Geometry: final body of the model. Coordinates: model frame, mm. A direction names the side the tool comes from. Coordinates: 2 decimals unless noted, no trailing zeros. Order: outer loops, then holes, each group sorted by start corner. A loop starts at its lowest first (then second) coordinate and runs counter-clockwise, first axis right, second up. Notation, with made-up numbers: (77, 32.25) -> (86, 32.25) arc R19 cw to (86, 38.25) -> close; hole circle Ø10 at (-26.5, 74.25). An arc over 180 degrees is marked (long way). Answer in a Markdown table with one row per item. Add a question column.
1) Section query A-A on y = 19.5. Return the cut outline in (x, z).
2) Contact query for flat-ended pins moving along their axis: P1, Ø8, axis at x = 9, z = 41.5, coming from the +Y side; P2, Ø11, axis at x = 16, z = 33.5, coming from the -Y side; P3, Ø2, axis at x = 10, y = 4.5, coming from the -Z side. Output: stop coordinate, or through.
3) Set-up query: faces 1 (the face through (11.63, -2.46, 38.1)), 2 (the face through (11, 2, 23)), 3 (the face through (21.5, 14, 24)). Return all of +Z, -Z, +X, -X, +Y, -Y with unobstructed straight access to the full face (end or side cutting, diameter ignored); none if empty.
4) Ray query, line 1 (X direction, y = 17.5, z = 27); line 2 (Y direction, x = 9, z = 37); line 3 (Z direction, x = 9.25, y = 21). Return the intervals inside material, ascending. Write a range as from..to.
5) Pull-direction query (Z, two-part tool) for faces 4 (the face through (1, 12, 0)), 5 (the face through (11.63, -2.46, 8.1)), 6 (the face through (11, 14, 48.5)), 7 (the face through (11, -5, 9)); classes: +Z half, -Z half, draft (parallel to the pull), parting line (faces both ways), or undercut.
6) Section query D-D on x = 3. Return the cut outline in (y, z).
7) Section query B-B on x = 10.75. Return the cut outline in (y, z), then the cut area to 3 significant figures.
8) Section query C-C on z = 39.25. Return the cut outline in (x, y).
```python
from build123d import *

# Parameters (mm, degrees)
SKETCH2_W           = 21.5
SKETCH2_H           = 28.5
BOSS_EXTRUDE6_DEPTH = 48.5
CUT_EXTRUDE5_DEPTH  = 46.5
SKETCH5_R           = 1.45
BOSS_EXTRUDE7_DEPTH = 5


with BuildPart() as part:
    # Sketch2 → Boss-Extrude6 (new body)
    with BuildSketch(Plane.XY):
        with Locations((10.75, 14.25)):
            Rectangle(SKETCH2_W, SKETCH2_H)
    extrude(amount=BOSS_EXTRUDE6_DEPTH)

    # 3DSketch6 → Cut-Extrude5 (cut)
    with BuildSketch(Plane(origin=(19.5, 2, 0), x_dir=(-0.5510615347417098, 0.8344646097517326, 0), z_dir=(0, 0, 1))):
        Polygon((0, 0), (22.113312158, -14.603130671), (31.756889016, 0), (9.643576858, 14.603130671), align=None)
    extrude(amount=CUT_EXTRUDE5_DEPTH, mode=Mode.SUBTRACT)

    # Sketch5 → Boss-Extrude7 (add)
    with BuildSketch(Plane(origin=(0, 0, 0), x_dir=(-1, 0, 0), z_dir=(0, -1, 0))):
        with Locations(Location((-10.75, -39.25, 0), (0, 0, 270))):
            Circle(SKETCH5_R)
        with Locations(Location((-10.75, -9.25, 0), (0, 0, 270))):
            Circle(SKETCH5_R)
    extrude(amount=BOSS_EXTRUDE7_DEPTH)


solid = part.part
```
Result:
| question | item | result |
|---|---|---|
| 1 | outline | (0, 0) -> (2, 0) -> (2, 46.5) -> (19.5, 46.5) -> (19.5, 0) -> (21.5, 0) -> (21.5, 48.5) -> (0, 48.5) -> close |
| 2 | P1 | y = 2 |
| 2 | P2 | y = 0 |
| 2 | P3 | z = 46.5 |
| 3 | face 1 | -Y |
| 3 | face 2 | -Z, +Y |
| 3 | face 3 | +Z, -Z, +X, +Y, -Y |
| 4 | line 1 | 0..2, 19.5..21.5 |
| 4 | line 2 | 0..2 |
| 4 | line 3 | 46.5..48.5 |
| 5 | face 4 | -Z half |
| 5 | face 5 | undercut |
| 5 | face 6 | +Z half |
| 5 | face 7 | draft |
| 6 | outline | (0, 0) -> (2, 0) -> (2, 46.5) -> (28.5, 46.5) -> (28.5, 48.5) -> (0, 48.5) -> close |
| 7 | outline | (-5, 7.8) -> (0, 7.8) -> (0, 0) -> (2, 0) -> (2, 46.5) -> (28.5, 46.5) -> (28.5, 48.5) -> (0, 48.5) -> (0, 40.7) -> (-5, 40.7) -> (-5, 37.8) -> (0, 37.8) -> (0, 10.7) -> (-5, 10.7) -> close |
| 7 | area | 179 mm2 |
| 8 | outline | (0, 0) -> (9.3, 0) -> (9.3, -5) -> (12.2, -5) -> (12.2, 0) -> (21.5, 0) -> (21.5, 28.5) -> (19.5, 28.5) -> (19.5, 2) -> (2, 2) -> (2, 28.5) -> (0, 28.5) -> close |
